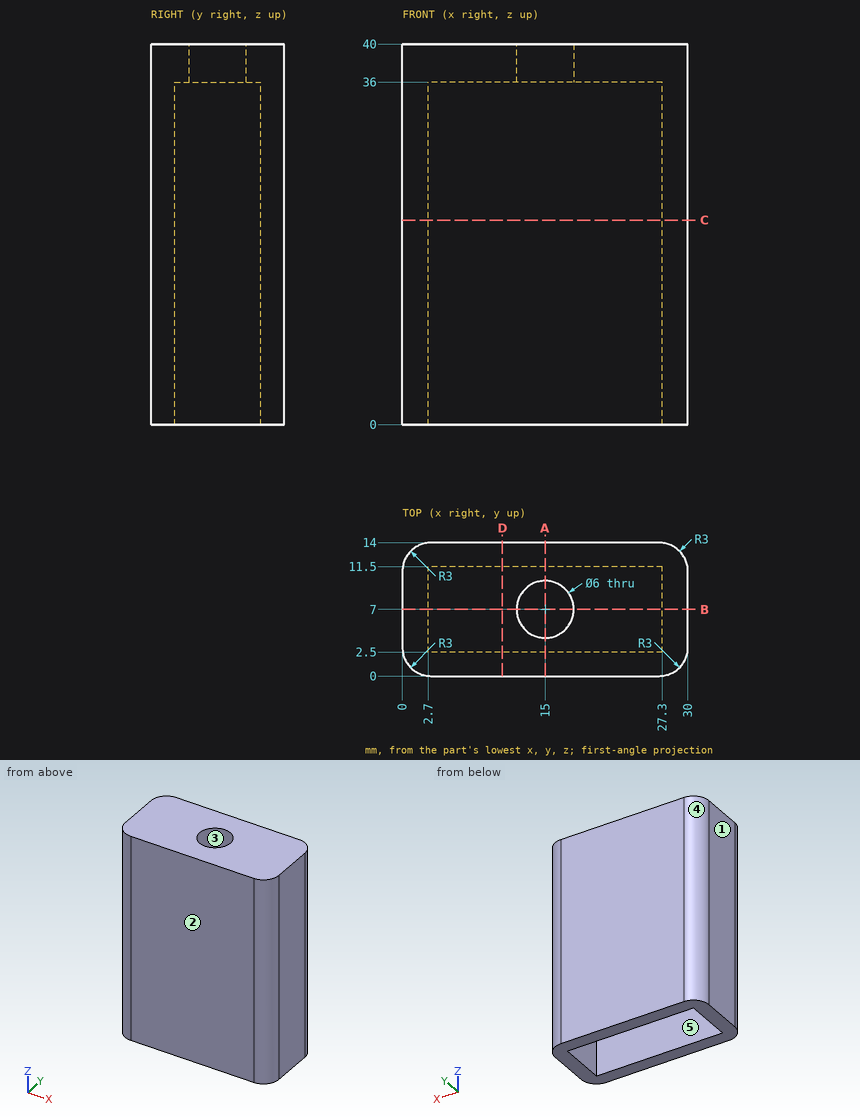
Design review of the part shown in the three views and the two pictorial views. Dimensions are in mm from the part's minimum x, y and z. A direction names the side the tool comes from. Round coordinates to 2 decimals unless told otherwise and drop trailing zeros. Order: outer loops, then holes, each group sorted by start corner. A loop starts at its lowest first (then second) coordinate and runs counter-clockwise, first axis right, second up.
(1) Take a section at C-C, the plane z = 21.5. State the section outline as (x, y) points, plus the area to 3 significant figures.
Working result:
outline: (0, 3) arc R3 ccw to (3, 0) - (27, 0) arc R3 ccw to (30, 3) - (30, 11) arc R3 ccw to (27, 14) - (3, 14) arc R3 ccw to (0, 11) - close; hole (2.7, 2.5) - (27.3, 2.5) - (27.3, 11.5) - (2.7, 11.5) - close
area: 191 mm2
(2) Take a section at B-B, the plane y = 7. State the section outline as (x, z) points, plus the area to 3 significant figures.
Working result:
outline: (0, 0) - (2.7, 0) - (2.7, 36) - (12, 36) - (12, 40) - (0, 40) - close; (18, 36) - (27.3, 36) - (27.3, 0) - (30, 0) - (30, 40) - (18, 40) - close
area: 290 mm2
(3) Wall thickness on L1, parallel to Y at x = 9, z = 33; L2, parallel to Y at x = 15, z = 36.9; L3, parallel to X at y = 7.5, z = 31: over which ranges is each line inside the solid? List them lowest first.
Working result:
L1: y = 0 to 2.5, 11.5 to 14
L2: y = 0 to 4, 10 to 14
L3: x = 0 to 2.7, 27.3 to 30
(4) Mouldability with a two-part tool opening along Y and no side actions: class the marked faces 1, 2 and 3 as released by +Y, released by -Y, zero draft, split by the parting line, or undercut.
Working result:
face 1: zero draft
face 2: released by -Y
face 3: undercut
(5) Take a section at A-A, the plane x = 15. State the section outline as (y, z) points, plus the area to 3 significant figures.
Working result:
outline: (0, 0) - (2.5, 0) - (2.5, 36) - (4, 36) - (4, 40) - (0, 40) - close; (10, 36) - (11.5, 36) - (11.5, 0) - (14, 0) - (14, 40) - (10, 40) - close
area: 212 mm2
(6) Tool access review of the marked faces 4 and 5: name each direction out of +Z, -Z, +X, -X, +Y, -Y from which nothing blocks a thin tool from reaching the whole face with its end or side.
Working result:
face 4: +Z, -Z, -X, +Y
face 5: -Z
(7) For P1, Ø7, axis at x = 15, y = 7, coming from the -Z side, flat-tipped, find the tip position at first contact; note if it passes through.
Working result:
P1: stops at z = 36
(8) Take a section at D-D, the plane x = 10.5. State the section outline as (y, z) points, plus the area to 3 significant figures.
Working result:
outline: (0, 0) - (2.5, 0) - (2.5, 36) - (11.5, 36) - (11.5, 0) - (14, 0) - (14, 40) - (0, 40) - close
area: 236 mm2
